Build history of the part. All positions in model axes, mm. A direction names the side the tool comes from. Round coordinates to 2 decimals unless told otherwise and drop trailing zeros. Write each loop counter-clockwise with the first axis right and the second up, starting at its lowest first coordinate (ties: lowest second). Pieces come first, ordered by that corner, then holes. Notation, with made-up numbers: M 28,-28.5 L 33,-28.5 A28 ccw 33,-5.5 Z; hole C 24,-4 d10. An arc over 180 degrees is marked long. Use a Markdown table: item, result.
from build123d import *

# Parameters (mm, degrees)
F0_W           = 55
F0_H           = 42
F1_DEPTH       = 15
F3_DEPTH       = 8
F4_DEPTH       = 14
F4_DEPTH_BACK  = 3
F6_D           = 7
F6_CSINK_D     = 10
F6_CSINK_ANGLE = 90
F7_R           = 5


# Not quite as in the source:
# - a pattern or mirror of a feature is missing from the dataset's text; its kind, count and spacing are read off the source's solid


with BuildPart() as f1:
    # F0 (on Front) → F1 (new body)
    with BuildSketch(Plane.XZ):
        with Locations((0, -21)):
            Rectangle(F0_W, F0_H)
    extrude(amount=-F1_DEPTH)

    # F2 (on face) → F3 (join)
    with BuildSketch(Plane.YZ.offset(27.5)):
        with BuildLine():
            Line((0, -42), (0, -21.960586854))
            Line((0, -21.960586854), (-26.9221419573, -47.7830788612))
            ThreePointArc((-26.9221419573, -47.7830788612), (-16.0770814164, -45.8015919972), (-10, -55))
            ThreePointArc((-10, -55), (-10.8015919972, -58.9229185836), (-13.0778580427, -62.2169211388))
            Line((-13.0778580427, -62.2169211388), (8, -42))
            Line((8, -42), (0, -42))
        make_face()
    f3 = extrude(amount=-F3_DEPTH)

    # F3_copies: F3 across plane
    add(f3.mirror(Plane(origin=(0, 0, 0), x_dir=(0, 0, -1), z_dir=(-1, 0, 0))))

    # F2 (on face) → F4 (join, two sides)
    with BuildSketch(Plane.YZ.offset(27.5)) as f4_sk:
        with BuildLine():
            ThreePointArc((-10, -55), (-16.0770814164, -45.8015919972), (-26.9221419573, -47.7830788612))
            Line((-26.9221419573, -47.7830788612), (-23.4610709786, -51.3915394306))
            ThreePointArc((-23.4610709786, -51.3915394306), (-18.0385407082, -50.4007959986), (-15, -55))
            ThreePointArc((-15, -55), (-15.4007959986, -56.9614592918), (-16.5389290214, -58.6084605694))
            Line((-16.5389290214, -58.6084605694), (-13.0778580427, -62.2169211388))
            ThreePointArc((-13.0778580427, -62.2169211388), (-10.8015919972, -58.9229185836), (-10, -55))
        make_face()
        with BuildLine():
            Line((-23.4610709786, -51.3915394306), (-26.9221419573, -47.7830788612))
            ThreePointArc((-26.9221419573, -47.7830788612), (-27.2169211388, -61.9221419573), (-13.0778580427, -62.2169211388))
            Line((-13.0778580427, -62.2169211388), (-16.5389290214, -58.6084605694))
            ThreePointArc((-16.5389290214, -58.6084605694), (-23.6084605694, -58.4610709786), (-23.4610709786, -51.3915394306))
        make_face()
    f4 = extrude(amount=-F4_DEPTH) + extrude(f4_sk.sketch, amount=F4_DEPTH_BACK)

    # F4_copies: F4 across plane
    add(f4.mirror(Plane(origin=(0, 0, 0), x_dir=(0, 0, -1), z_dir=(-1, 0, 0))))

    # F6 (through all)
    with Locations(Plane.XZ):
        with Locations((-15, -10), (0, -30)):
            f6 = CounterSinkHole(F6_D / 2, F6_CSINK_D / 2, counter_sink_angle=F6_CSINK_ANGLE)

    # F6_copies: F6 across plane
    add(f6.mirror(Plane(origin=(0, 0, 0), x_dir=(0, 0, 1), z_dir=(1, 0, 0))), mode=Mode.SUBTRACT)

    # F7
    f7_edges = [f1.edges().sort_by_distance(p)[0] for p in [
        (27.5, 7.5, 0),
    ]]
    fillet(f7_edges, radius=F7_R)


solid = f1.part
Q1. Two-plate mould, pull along X, no slides. Class faces 4 (the conical face through (4, 1, -30)), 5 (the flat face through (27.5, -2, -33)), 6 (the flat face through (-19.5, -7, -41)), 7 (the flat face through (-23.56, -13.27, -34.69)): +X half, -X half, draft (parallel to the pull), parting line (faces both ways), or undercut.
Response values:
| item | result |
|---|---|
| face 4 | undercut |
| face 5 | +X half |
| face 6 | undercut |
| face 7 | draft |
Q2. Which spindle directions (+Z, -Z, +X, -X, +Y, -Y) get a long thin tool onto all of the face, cutting with end or side? Do faces 1 (the flat face through (13.5, -18, -50)), 2 (the flat face through (0, 0, -21)), 3 (the conical face through (15, 1, -6)). Say none if no direction does.
Response values:
| item | result |
|---|---|
| face 1 | +Z, -Z, +Y, -Y |
| face 2 | +Z, -Y |
| face 3 | -Y |
Q3. Cut at A-A on x = -15. Give the cut face in (y, z).
Response values:
| item | result |
|---|---|
| outline | C -20,-55 d20; M 0,-42 L 15,-42 L 15,-13.5 L 1.5,-13.5 L 0,-15 Z; M 0,-5 L 1.5,-6.5 L 15,-6.5 L 15,0 L 0,0 Z; hole C -20,-55 d10 |
Q4. Drop flat-ended pins along their axis: P1, Ø12.5, axis at y = -12.5, z = -39, coming from the +X side; P2, Ø4, axis at x = -15, z = -10, coming from the -Y side; P3, Ø4.5, axis at x = 13, y = 5.5, coming from the -Z side; P4, Ø12.5, axis at y = -0.5, z = -44, coming from the -X side. Give the stop position or say it passes through.
Response values:
| item | result |
|---|---|
| P1 | stops at x = 27.5 |
| P2 | passes through |
| P3 | stops at z = -42 |
| P4 | stops at x = -27.5 |
Q5. Drill centre lines: L1, parallel to X at y = 8.25, z = -10; L2, parallel to Z at x = 28.5, y = -20; L3, parallel to Z at x = -15, y = 6.5. Where is each one in solid material? Low to high.
Response values:
| item | result |
|---|---|
| L1 | x = -27.5 to -18.5, -11.5 to 11.5, 18.5 to 27.5 |
| L2 | z = -65 to -60, -50 to -45 |
| L3 | z = -42 to -13.5, -6.5 to 0 |
Q6. Cut at B-B on y = 11.5. Give the cut face in (x, z), and give its area (3 significant figures).
Response values:
| item | result |
|---|---|
| outline | M -27.5,-42 L 27.5,-42 L 27.5,-5 A5 ccw 22.5,0 L -27.5,0 Z; hole C -15,-10 d7; hole C 0,-30 d7; hole C 15,-10 d7 |
| area | 2,190 mm2 |
Q7. Cut at D-D on y = -18. Give the cut face in (x, z), and give its area (3 significant figures).
Response values:
| item | result |
|---|---|
| outline | M -30.5,-64.8 L -13.5,-64.8 L -13.5,-59.58 L -30.5,-59.58 Z; M -30.5,-50.42 L -13.5,-50.42 L -13.5,-45.2 L -19.5,-45.2 L -19.5,-39.23 L -27.5,-39.23 L -27.5,-45.2 L -30.5,-45.2 Z; M 13.5,-64.8 L 30.5,-64.8 L 30.5,-59.58 L 13.5,-59.58 Z; M 13.5,-50.42 L 30.5,-50.42 L 30.5,-45.2 L 27.5,-45.2 L 27.5,-39.23 L 19.5,-39.23 L 19.5,-45.2 L 13.5,-45.2 Z |
| area | 450 mm2 |
Q8. Cut at C-C on x = 0. Give the cut face in (y, z).
Response values:
| item | result |
|---|---|
| outline | M 0,-42 L 15,-42 L 15,-33.5 L 1.5,-33.5 L 0,-35 Z; M 0,-25 L 1.5,-26.5 L 15,-26.5 L 15,0 L 0,0 Z |
